For this review, use the dimensioned drawing (mm, ordinates from the lowest corner) and the shaded views. Round coordinates to 2 decimals unless told otherwise and drop trailing zeros. Order: outer loops, then holes, each group sorted by start corner. A loop starts at its lowest first (then second) coordinate and runs counter-clockwise, first axis right, second up. Notation, with made-up numbers: M 1,-3 L 28,-3 A23 ccw 28,7 Z; hole C 52,87 d5. An arc over 180 degrees is marked long. Use a Markdown table: item, result. Add a question column.
1. Insertion check: P1, Ø1.2, axis at x = 1, z = 2, coming from the +Y side; P2, Ø2, axis at y = 9, z = 41, coming from the -X side; P3, Ø1.2, axis at x = 1, z = 2, coming from the -Y side; P4, Ø0.8, axis at x = 1.5, y = 15.5, coming from the +Z side. Each pin has a flat end and moves straight along its axis. Give the tip position at first contact, or say it passes through.
2. To check wall thickness, follow probe 1 along Z at (x, y) = (0.8, 1.25). State the ranges of the line that lie inside material, in increasing order.
3. Consider section A-A on x = 1.25. State the section outline as (y, z) points.
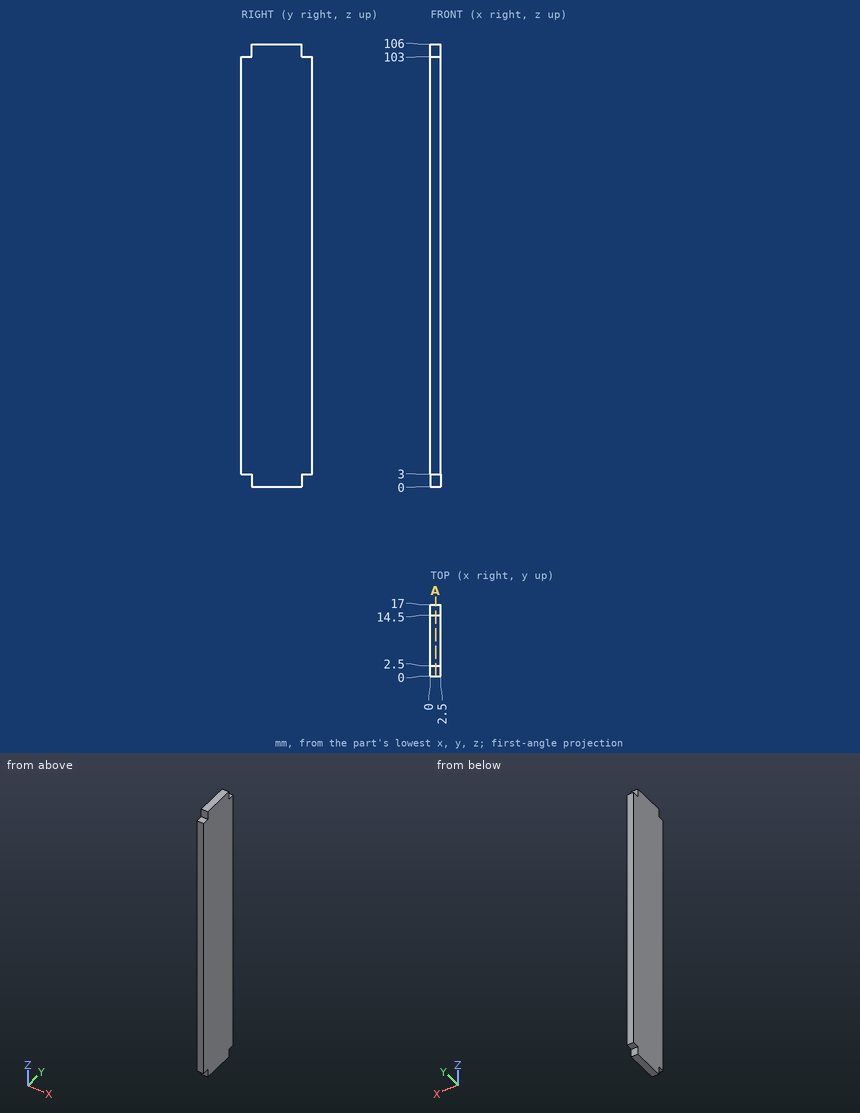
Answer block:
| question | item | result |
|---|---|---|
| 1 | P1 | y = 14.5 |
| 1 | P2 | x = 0 |
| 1 | P3 | y = 2.5 |
| 1 | P4 | z = 103 |
| 2 | probe 1 | 3 to 103 |
| 3 | outline | M 0,3 L 2.5,3 L 2.5,0 L 14.5,0 L 14.5,3 L 17,3 L 17,103 L 14.5,103 L 14.5,106 L 2.5,106 L 2.5,103 L 0,103 Z |
